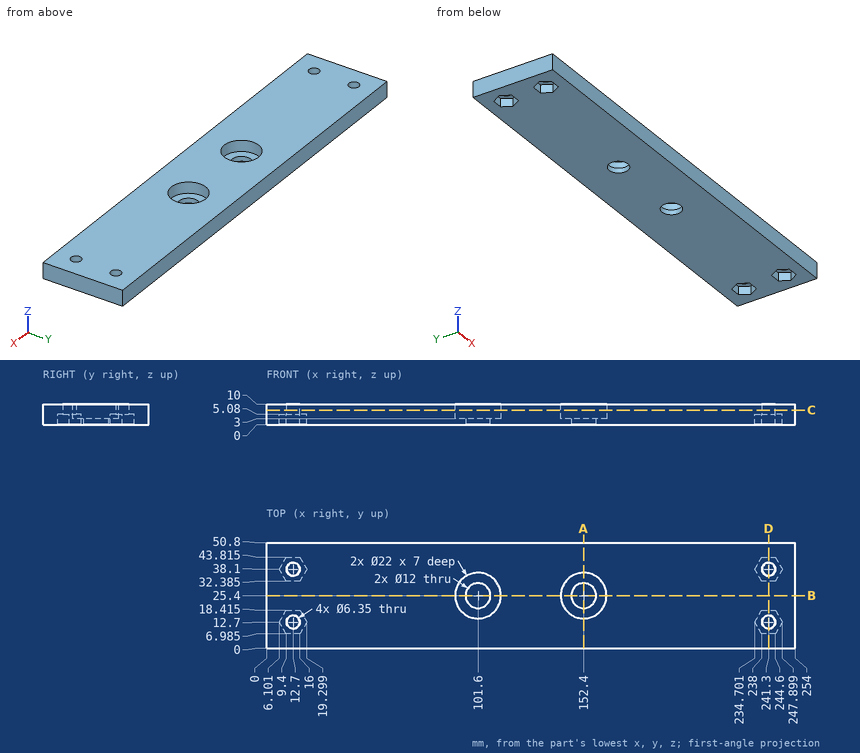
Here's the drawing with two shaded views (mm, measured from the low corner). I have some questions. Coordinates: 2 decimals unless noted, no trailing zeros. Write each loop counter-clockwise with the first axis right and the second up, starting at its lowest first coordinate (ties: lowest second). Pieces come first, ordered by that corner, then holes.
Item 1: I want a section at B-B on y = 25.4. Write out the boundary of the cut face in (x, z).
Item 2: If I drill on line 1 (Y direction, x = 12.7, z = 8.55) (1 decimal); line 2 (X direction, y = 25.5, z = 7.75); line 3 (X direction, y = 25.5, z = 2.75), over which ranges is the centre line in solid material (lowest first)?
Item 3: I want a section at C-C on z = 7. Count the separate pieces of the cut face and the enclosed holes in it, and give its area (3 significant figures).
Item 4: I want a section at D-D on x = 241.3. Write out the boundary of the cut face in (y, z) (1 decimal).
Item 5: I want a section at A-A on x = 152.4. Write out the boundary of the cut face in (y, z), and give its area (3 significant figures).
Item 6: Will these pins go through, and if not, where does the flat tip stop? pin 1 (9 mm diameter, centred on x = 12.5, y = 12.5, fed in from -Z); pin 2 (17.5 mm diameter, centred on x = 101.6, y = 25.4, fed in from +Z); pin 3 (1.5 mm diameter, centred on x = 12.5, z = 3.5, fed in from -Y).
Findings below:
1. outline: (0, 0) - (95.6, 0) - (95.6, 3) - (90.6, 3) - (90.6, 10) - (0, 10) - close; (107.6, 0) - (146.4, 0) - (146.4, 3) - (141.4, 3) - (141.4, 10) - (112.6, 10) - (112.6, 3) - (107.6, 3) - close; (158.4, 0) - (254, 0) - (254, 10) - (163.4, 10) - (163.4, 3) - (158.4, 3) - close
2. line 1: y = 0 to 9.5, 15.9 to 34.9, 41.3 to 50.8
2. line 2: x = 0 to 90.6, 112.6 to 141.4, 163.4 to 254
2. line 3: x = 0 to 95.6, 107.6 to 146.4, 158.4 to 254
3. separate pieces: 1
3. enclosed holes: 6
3. area: 12,000 mm2
4. outline: (0, 0) - (7, 0) - (7, 5.1) - (9.5, 5.1) - (9.5, 10) - (0, 10) - close; (15.9, 5.1) - (18.4, 5.1) - (18.4, 0) - (32.4, 0) - (32.4, 5.1) - (34.9, 5.1) - (34.9, 10) - (15.9, 10) - close; (41.3, 5.1) - (43.8, 5.1) - (43.8, 0) - (50.8, 0) - (50.8, 10) - (41.3, 10) - close
5. outline: (0, 0) - (19.4, 0) - (19.4, 3) - (14.4, 3) - (14.4, 10) - (0, 10) - close; (31.4, 0) - (50.8, 0) - (50.8, 10) - (36.4, 10) - (36.4, 3) - (31.4, 3) - close
5. area: 318 mm2
6. pin 1: stops at z = 5.08
6. pin 2: stops at z = 3
6. pin 3: stops at y = 0
